from build123d import *

# Parameters (mm, degrees)
F0_W     = 50.8
F0_H     = 4.7625
F1_DEPTH = 15.875
F0_R     = 1.5875
F2_DEPTH = 4.7625
F4_DEPTH = 25.4


with BuildPart() as f1:
    # F0 (on Top) → F1 (new body)
    with BuildSketch(Plane.XY):
        with Locations((25.4, 2.38125)):
            Rectangle(F0_W, F0_H)
    extrude(amount=F1_DEPTH)

    # F0 (on Top) → F2 (join)
    with BuildSketch(Plane.XY):
        with Locations((25.4, 2.38125)):
            Rectangle(F0_W, F0_H)
        with BuildLine():
            Line((0, 38.1), (0, 4.7625))
            Line((0, 4.7625), (50.8, 4.7625))
            Line((50.8, 4.7625), (50.8, 38.1))
            ThreePointArc((50.8, 38.1), (48.940128, 42.590128), (44.45, 44.45))
            Line((44.45, 44.45), (6.35, 44.45))
            ThreePointArc((6.35, 44.45), (1.859872, 42.590128), (0, 38.1))
        make_face()
        with Locations((15.875, 15.875)):
            Circle(F0_R, mode=Mode.SUBTRACT)
        with Locations((34.925, 15.875)):
            Circle(F0_R, mode=Mode.SUBTRACT)
        with Locations((6.35, 38.1)):
            Circle(F0_R, mode=Mode.SUBTRACT)
        with Locations((44.45, 38.1)):
            Circle(F0_R, mode=Mode.SUBTRACT)
    extrude(amount=F2_DEPTH)

    # F3 (on face) → F4 (cut)
    with BuildSketch(Plane.XZ):
        with BuildLine():
            ThreePointArc((0, 9.525), (1.859872, 14.015128), (6.35, 15.875))
            Line((6.35, 15.875), (0, 15.875))
            Line((0, 15.875), (0, 9.525))
        make_face()
        with BuildLine():
            ThreePointArc((4.7625, 9.525), (6.35, 7.9375), (7.9375, 9.525))
            ThreePointArc((7.9375, 9.525), (7.472532, 10.647532), (6.35, 11.1125))
            Line((6.35, 11.1125), (6.35, 9.525))
            Line((6.35, 9.525), (4.7625, 9.525))
        make_face()
        with BuildLine():
            Line((6.35, 9.525), (6.35, 11.1125))
            ThreePointArc((6.35, 11.1125), (5.227468, 10.647532), (4.7625, 9.525))
            Line((4.7625, 9.525), (6.35, 9.525))
        make_face()
        with BuildLine():
            Line((50.8, 15.875), (44.45, 15.875))
            ThreePointArc((44.45, 15.875), (48.940128, 14.015128), (50.8, 9.525))
            Line((50.8, 9.525), (50.8, 15.875))
        make_face()
        with BuildLine():
            ThreePointArc((46.0375, 9.525), (45.572532, 10.647532), (44.45, 11.1125))
            Line((44.45, 11.1125), (44.45, 9.525))
            Line((44.45, 9.525), (46.0375, 9.525))
        make_face()
        with BuildLine():
            Line((44.45, 9.525), (44.45, 11.1125))
            ThreePointArc((44.45, 11.1125), (43.327468, 8.402468), (46.0375, 9.525))
            Line((46.0375, 9.525), (44.45, 9.525))
        make_face()
    extrude(amount=-F4_DEPTH, mode=Mode.SUBTRACT)


solid = f1.part
CAD build for the part. Positions are in the model's coordinates, mm. A direction names the side the tool comes from. Round coordinates to 2 decimals unless told otherwise and drop trailing zeros. Order: outer loops, then holes, each group sorted by start corner. A loop starts at its lowest first (then second) coordinate and runs counter-clockwise, first axis right, second up. Notation, with made-up numbers: (42, 20) - (99, 20) arc R20 cw to (99, 40) - close; hole circle Ø9 at (57.25, 29). An arc over 180 degrees is marked (long way). Return JSON: item names as keys, results as strings.
(1) Pin check, flat tips, straight feed: pin 1 Ø6 at (x, y) = (16.5, 33.5) entering from +Z; pin 2 Ø5.5 at (x, z) = (22.5, 10.5) entering from +Y. Stop position of each tip, or through.
Answer key:
{"pin 1": "stops at z = 4.76", "pin 2": "stops at y = 4.76"}
(2) Cut at A-A (z = 4). State how many separate pieces and enclosed holes the cut face has, then the cut area to 3 significant figures.
Answer key:
{"separate pieces": "1", "enclosed holes": "4", "area": "2,210 mm^2"}
(3) Cut at C-C (y = 29.5). Give the cut face in (x, z), then the cut area to 3 significant figures.
Answer key:
{"outline": "(0, 0) - (50.8, 0) - (50.8, 4.76) - (0, 4.76) - close", "area": "242 mm^2"}
(4) Tool access for faces 1 (the face through (25, 4.762, 10)), 2 (the face through (1.811, 2.348, 13.965)): list every direction of +Z, -Z, +X, -X, +Y, -Y with a clear straight run to the whole face (end or side of a thin tool).
Answer key:
{"face 1": "+Z, +X, -X, +Y", "face 2": "+Z, -X, +Y, -Y"}
(5) Wall check: probe 1 along Y at (x, z) = (44.45, 1.1); probe 2 along Z at (x, y) = (45.5, 10). Give the ranges that are in metal, low to high. Write a range as from..to.
Answer key:
{"probe 1": "y = 0..36.51, 39.69..44.45", "probe 2": "z = 0..4.76"}
(6) Pull direction X, two halves, no side cores. Call faces 3 (the face through (0, 19, 3)), 4 (the face through (15.531, 14.325, 2.348)), 5 (the face through (48.89, 2.348, 14.064)), 6 (the face through (26, 44.45, 2)): +X half, -X half, draft (parallel to the pull), parting line (faces both ways), or undercut.
Answer key:
{"face 3": "-X half", "face 4": "undercut", "face 5": "+X half", "face 6": "draft"}
